Input: part model. Units: mm. Frame: model coordinates. Face numbers are marked on the shaded views. A direction names the side the tool comes from. Coordinates: 2 decimals unless noted, no trailing zeros. Write each loop counter-clockwise with the first axis right and the second up, starting at its lowest first coordinate (ties: lowest second). Pieces come first, ordered by that corner, then holes. Notation, with made-up numbers: (65.25, -9.75) - (69.25, -9.75) arc R19 ccw to (69.25, 18.25) - close; hole circle Ø1 at (-22, 66.25). An arc over 180 degrees is marked (long way). Use CSV: the item, a comma, the result in double quotes.
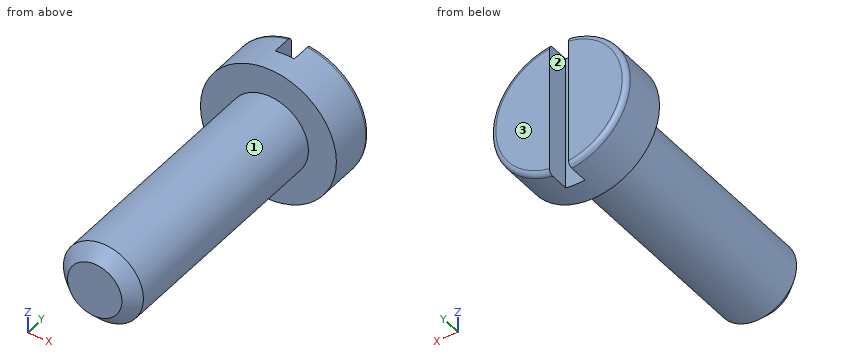
```python
from build123d import *

# Parameters (mm, degrees)
TIGE_START              = -16
ESQUISSE1_R             = 2.5
TIGE_DEPTH              = 16
CHANFREIN_D_ENTR_E_SIZE = 0.8
ESQUISSE3_W             = 1.2
ESQUISSE3_H             = 8.5
FENTE_DEPTH             = 1.5


with BuildPart() as part:
    # Esquisse1 → Tige (new body)
    with BuildSketch(Plane(origin=(0, 0, 0), x_dir=(1, 0, 0), z_dir=(0, 1, 0)).offset(TIGE_START)):
        with Locations(Location((0, 0, 0), (0, 0, 270))):
            Circle(ESQUISSE1_R)
    extrude(amount=TIGE_DEPTH)

    # Chanfrein d'entrée
    chanfrein_d_entr_e_edges = [part.edges().sort_by_distance(p)[0] for p in [
        (0, -16, -2.5),
    ]]
    chamfer(chanfrein_d_entr_e_edges, length=CHANFREIN_D_ENTR_E_SIZE)

    # Esquisse2 → Tête (revolve)
    with BuildSketch(Plane.XY, mode=Mode.PRIVATE) as t_te_sk:
        with BuildLine():
            Line((0, 0), (4.25, 0))
            Line((4.25, 0), (4.25, 2.7))
            ThreePointArc((4.25, 2.7), (4.162132034, 2.912132034), (3.95, 3))
            Line((3.95, 3), (0, 3))
            Line((0, 3), (0, 0))
        make_face()
    revolve(t_te_sk.sketch.rotate(Axis((0, 3, 0), (0, -1, 0)), 180), axis=Axis((0, 3, 0), (0, -1, 0)))

    # Esquisse3 → Fente (cut)
    with BuildSketch(Plane(origin=(0, 3, -1.8), x_dir=(1, 0, 0), z_dir=(0, -1, 0))):
        with Locations((0, 1.8)):
            Rectangle(ESQUISSE3_W, ESQUISSE3_H)
    extrude(amount=FENTE_DEPTH, mode=Mode.SUBTRACT)


solid = part.part
```
(1) Cut plane D-D on y = 0.5. Return loops of the section in (x, z), and give its area (3 significant figures).
Check values:
outline,"circle Ø8.5 at (0, 0)"
area,"56.7 mm^2"
(2) Cut plane A-A on x = 0. Return loops of the section in (y, z), and give its area (3 significant figures).
Check values:
outline,"(-16, -1.7) - (-15.2, -2.5) - (0, -2.5) - (0, -4.25) - (1.5, -4.25) - (1.5, 4.25) - (0, 4.25) - (0, 2.5) - (-15.2, 2.5) - (-16, 1.7) - close"
area,"92.1 mm^2"
(3) Ray query, probe 1 along Y at (x, z) = (2.75, -1); probe 2 along Z at (x, y) = (2, -2.5); probe 3 along Z at (x, y) = (-0.25, -12). Return the intervals inside material, ascending. Write a range as from..to.
Check values:
probe 1,"0..3"
probe 2,"-1.5..1.5"
probe 3,"-2.49..2.49"
(4) Cut plane C-C on y = -8. Return loops of the section in (x, z).
Check values:
outline,"circle Ø5 at (0, 0)"
(5) Reachability of the marked faces 1, 2 and 3 from +Z, -Z, +X, -X, +Y, -Y: full face, straight path, thin tool, end or side. Return the list, or none.
Check values:
face 1,"-Y"
face 2,"+Z, -Z, +Y"
face 3,"+Z, -Z, +X, -X, +Y"
(6) Pin query (flat end, axial travel): pin 1 Ø1 at (x, y) = (2.5, -4) entering from +Z; pin 2 Ø1.7 at (y, z) = (2.5, 1) entering from -X; pin 3 Ø3 at (y, z) = (-7.5, 2.5) entering from -X. Return the tip coordinate at first contact, or that it passes through.
Check values:
pin 1,"z = 1.5"
pin 2,"x = -4.25"
pin 3,"x = -2.29"
(7) Cut plane B-B on z = 0. Return loops of the section in (x, y), and give its area (3 significant figures).
Check values:
outline,"(-4.25, 0) - (-2.5, 0) - (-2.5, -15.2) - (-1.7, -16) - (1.7, -16) - (2.5, -15.2) - (2.5, 0) - (4.25, 0) - (4.25, 2.7) arc R0.3 ccw to (3.95, 3) - (0.6, 3) - (0.6, 1.5) - (-0.6, 1.5) - (-0.6, 3) - (-3.95, 3) arc R0.3 ccw to (-4.25, 2.7) - close"
area,"103 mm^2"
